Autodesk Inventor part; units mm, degrees
ref_plane "YZ Plane" through (0, 0, 0) normal (1, 0, 0) x (0, 1, 0)
ref_plane "XZ Plane" through (0, 0, 0) normal (0, 1, 0) x (-1, 0, 0)
ref_plane "XY Plane" through (0, 0, 0) normal (0, 0, 1) x (1, 0, 0)
sketch "Sketch1" plane through (0, 0, 0) normal (0, 0, 1) x (1, 0, 0)
  line L0 (0, 0) -> (10, 0)
  line L1 (-2, 0) -> (12, 0) construction
  line L2 (0, 0) -> (0, 10)
  line L3 (10, 0) -> (10, 10)
  line L4 (0, 10) -> (10, 10)
  dimension "d0" = 10
  dimension "d1" = 10
  dimension "d2" = 10
extrude "Extrusion1" add sketch "Sketch1" along normal blind 10
sketch "Sketch2" plane through (10, 0, 0) normal (1, 0, 0) x (0, 0, -1)
  circle A0 centre (-5, 5) radius 1.5
  line L0 (-10, 0) -> (-10, 10)
  line L1 (0, 0) -> (-10, 0)
  point P0 (-10, 5)
  point P1 (-5, 0)
  dimension "d5" = 3
extrude "Extrusion2" cut sketch "Sketch2" against normal up to surface (10 mm away)
equation "\"d1\" = d0"
equation "\"d2\" = d1"
properties part number "01Cubo"
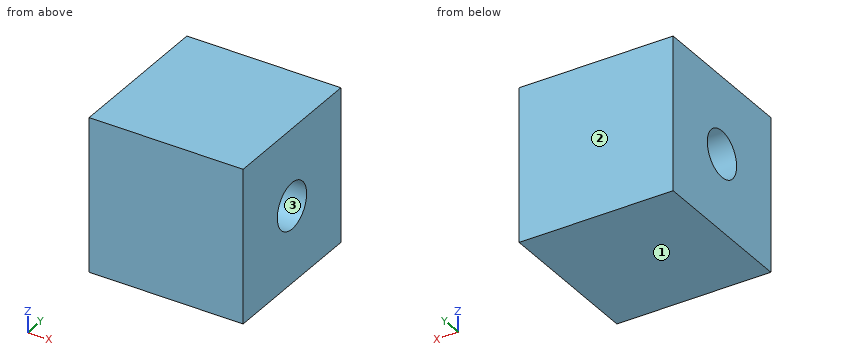
Design review of the part built by this model. Coordinates are the model's own, in mm. Face numbers are marked on the shaded views. Coordinates: 2 decimals unless noted, no trailing zeros. Order: outer loops, then holes, each group sorted by start corner. A loop starts at its lowest first (then second) coordinate and runs counter-clockwise, first axis right, second up. Notation, with made-up numbers: M 5,78 L 33,78 A24 ccw 33,90 Z; hole C 73.5,17.5 d1. An arc over 180 degrees is marked long. Answer as a JSON object with one key per item and string values. Group by question number.
1) Add section C-C, the plane x = 5.25. Write out the cut boundary in (y, z), then the cut area to 3 significant figures.
2) Mouldability with a two-part tool opening along Y and no side actions: class the marked faces 1, 2 and 3 as pulls with the +Y half, pulls with the -Y half, needs draft (parallel to the pull), parting line crosses it, or undercut.
3) For pin 1 (5 mm diameter, centred on y = 5, z = 5, fed in from +X), flat-tipped, find the tip position at first contact; note if it passes through.
4) Wall thickness on L1, parallel to Y at x = 5.25, z = 5; L2, parallel to Z at x = 2, y = 4.25; L3, parallel to Z at x = 7, y = 6.25: over which ranges is each line inside the solid? List them lowest first.
5) Add section A-A, the plane y = 5. Write out the cut boundary in (x, z), then the cut area to 3 significant figures.
Computed values:
{
 "1": {"outline": "M 0,0 L 10,0 L 10,10 L 0,10 Z; hole C 5,5 d3", "area": "92.9 mm^2"},
 "2": {"face 1": "needs draft", "face 2": "pulls with the +Y half", "face 3": "undercut"},
 "3": {"pin 1": "stops at x = 10"},
 "4": {"L1": "y = 0 to 3.5, 6.5 to 10", "L2": "z = 0 to 3.7, 6.3 to 10", "L3": "z = 0 to 4.17, 5.83 to 10"},
 "5": {"outline": "M 0,0 L 10,0 L 10,3.5 L 0,3.5 Z; M 0,6.5 L 10,6.5 L 10,10 L 0,10 Z", "area": "70.0 mm^2"}
}
